Work out the finished part from the listing and answer in its coordinate system (mm). A direction names the side the tool comes from. Coordinates: 2 decimals unless noted, no trailing zeros. Write each loop counter-clockwise with the first axis right and the second up, starting at its lowest first coordinate (ties: lowest second). Pieces come first, ordered by that corner, then holes. Notation, with made-up numbers: (-3, 3.5) - (34, 3.5) arc R31 ccw to (34, 29.5) - close; hole circle Ø5 at (23, -2). An arc over 180 degrees is marked (long way). One line per item, written item: value.
```python
from build123d import *

# Parameters (mm, degrees)
F2_R = 1.99999
F3_R = 2


# Not quite as in the source:
# - a fillet or chamfer is up to 0.001 mm smaller than in the source, because OpenCascade refuses the exact size


with BuildPart() as f1:
    # F0 (on Right) → F1 (revolve)
    with BuildSketch(Plane.YZ):
        with BuildLine():
            Line((-2, -4.5), (0, -4.5))
            Line((0, -4.5), (0, -2))
            Line((0, -2), (-14.007930782, -2.2))
            Line((-14.007930782, -2.2), (-14.007930782, -3))
            Line((-14.007930782, -3), (-28, -3.5))
            Line((-28, -3.5), (-28, -4.5))
            Line((-28, -4.5), (-14, -4.5))
            ThreePointArc((-14, -4.5), (-8, -3.5651046907), (-2, -4.5))
        make_face()
    revolve(axis=Axis((0, -15.99, 0), (0, -1, 0)))

    # F2 (radius 2 in the source; OpenCascade refuses exactly that, so slightly less here)
    f2_edges = [f1.edges().sort_by_distance(p)[0] for p in [
        (0, 0, 4.5),
    ]]
    fillet(f2_edges, radius=F2_R)

    # F3
    f3_edges = [f1.edges().sort_by_distance(p)[0] for p in [
        (0, -14, 4.5),
    ]]
    fillet(f3_edges, radius=F3_R)


solid = f1.part
```
Item 1: Section B-B, the plane y = -8.5 is taken. Determine the outline of the cut face in (x, z).
Evaluation:
outline: circle Ø7.14 at (0, 0); hole circle Ø4.24 at (0, 0)
Item 2: Consider probe 1 along Y at (x, z) = (2.25, 1); probe 2 along X at (y, z) = (-11.75, 1); probe 3 along X at (y, z) = (-16, 1). Determine where each line is inside the solid, lowest interval first.
Evaluation:
probe 1: y = -14.01 to 0
probe 2: x = -3.8 to -1.92, 1.92 to 3.8
probe 3: x = -4.39 to -2.9, 2.9 to 4.39
Item 3: Which of the six approach directions +Z, -Z, +X, -X, +Y, -Y give full straight-line access (tool end or side, diameter ignored) to faces 1 (the face through (2, -14.008, -2)), 2 (the face through (-4, -28, 0))?
Evaluation:
face 1: -Y
face 2: +Z, -Z, +X, -X, -Y
Item 4: Given pin 1 (2 mm diameter, centred on x = -0.5, y = -3.5, fed in from +Z); pin 2 (3 mm diameter, centred on x = -2, y = -22.5, fed in from -Z); pin 3 (5 mm diameter, centred on y = -12, z = -2.5, fed in from +X), each flat-ended and moving along its own axis, determine where each tip first touches the part or whether it passes through.
Evaluation:
pin 1: stops at z = 4.33
pin 2: stops at z = -4.47
pin 3: stops at x = 4.37
Item 5: Determine the mould class of faces 3 (the face through (4.46, -21.06, 0.59)), 4 (the face through (2, 0, 1)), 5 (the face through (0.631, -7.102, -2.004)) for opening direction X: +X half, -X half, draft (parallel to the pull), parting line (faces both ways), or undercut.
Evaluation:
face 3: parting line
face 4: draft
face 5: undercut
Item 6: Section A-A, the plane y = -23.5 is taken. Determine the outline of the cut face in (x, z).
Evaluation:
outline: circle Ø9 at (0, 0); hole circle Ø6.68 at (0, 0)
